Verification items for the finished model (mm, model axes). A direction names the side the tool comes from. Round coordinates to 2 decimals unless told otherwise and drop trailing zeros. Write each loop counter-clockwise with the first axis right and the second up, starting at its lowest first coordinate (ties: lowest second). Pieces come first, ordered by that corner, then holes. Notation, with made-up numbers: M 65,-16.75 L 72,-16.75 A36 ccw 72,19.25 Z; hole C 4,56 d6. An arc over 180 degrees is marked long. Use a Markdown table: item, result. Add a question column.
from build123d import *

# Parameters (mm, degrees)
BOSS_EXTRUDE1_DEPTH = 12
FILLET1_R           = 3
SKETCH4_R           = 0.5
CUT_EXTRUDE3_DEPTH  = 121.732141537
FILLET2_R           = 1
FILLET3_R           = 1
FILLET4_R           = 1
FILLET6_R           = 1
SKETCH2_R           = 2
CUT_EXTRUDE1_DEPTH  = 122.116679281
SKETCH6_R           = 2
CUT_EXTRUDE4_DEPTH  = 8
CUT_EXTRUDE5_DEPTH  = 3.25


with BuildPart() as part:
    # Sketch1 → Boss-Extrude1 (new, symmetric)
    with BuildSketch(Plane(origin=(-107.5, 40, 0), x_dir=(0, 0, -1), z_dir=(1, 0, 0))):
        Polygon((-6.7, -37), (-6.7, -40), (0, -40), (0, -26), (10, -26), (10, -34), (6, -34), (3, -43), (-9.7, -43), (-9.7, -37), align=None)
    extrude(amount=BOSS_EXTRUDE1_DEPTH, both=True)

    # Fillet1
    fillet1_edges = [part.edges().sort_by_distance(p)[0] for p in [
        (-107.5, -3, -3),
        (-107.5, -3, 9.7),
    ]]
    fillet(fillet1_edges, radius=FILLET1_R)

    # Sketch4 → Cut-Extrude3 (cut, through all)
    with BuildSketch(Plane(origin=(0, 0, 0), x_dir=(0, 0, -1), z_dir=(1, 0, 0))):
        with Locations((-6.7, 0)):
            Circle(SKETCH4_R)
        Circle(SKETCH4_R)
    extrude(amount=-CUT_EXTRUDE3_DEPTH, mode=Mode.SUBTRACT)

    # Fillet2
    fillet2_edges = [part.edges().sort_by_distance(p)[0] for p in [
        (-107.5, 0, 6.2),
        (-107.5, 0.5, 6.7),
        (-107.5, 0.5, 0),
        (-107.5, 0, 0.5),
    ]]
    fillet(fillet2_edges, radius=FILLET2_R)

    # Fillet3
    fillet3_edges = [part.edges().sort_by_distance(p)[0] for p in [
        (-107.5, 3, 6.7),
        (-107.5, 3, 9.7),
    ]]
    fillet(fillet3_edges, radius=FILLET3_R)

    # Fillet4
    fillet4_edges = [part.edges().sort_by_distance(p)[0] for p in [
        (-107.5, 14, 0),
        (-107.5, 14, -10),
    ]]
    fillet(fillet4_edges, radius=FILLET4_R)

    # Fillet6
    fillet6_edges = [part.edges().sort_by_distance(p)[0] for p in [
        (-107.5, 6, -10),
        (-107.5, 6, -6),
    ]]
    fillet(fillet6_edges, radius=FILLET6_R)

    # Sketch2 → Cut-Extrude1 (cut, through all)
    with BuildSketch(Plane.XZ.offset(-14)):
        with Locations(Location((-107.5, -5, 0), (0, 0, 41.156184936))):
            Circle(SKETCH2_R)
    extrude(amount=CUT_EXTRUDE1_DEPTH, mode=Mode.SUBTRACT)

    # Sketch6 → Cut-Extrude4 (cut)
    with BuildSketch(Plane(origin=(0, 0, -10), x_dir=(-1, 0, 0), z_dir=(0, 0, -1))):
        with Locations((115.5, 10)):
            Circle(SKETCH6_R)
        with Locations((99.5, 10)):
            Circle(SKETCH6_R)
    extrude(amount=-CUT_EXTRUDE4_DEPTH, mode=Mode.SUBTRACT)

    # Sketch7 → Cut-Extrude5 (cut, symmetric)
    with BuildSketch(Plane(origin=(-107.5, 40, 0), x_dir=(0, 0, -1), z_dir=(1, 0, 0))):
        Polygon((1.88130822, -30.5), (8.38130822, -30.5), (10, -30.5), (10, -43), (8.38130822, -43), (1.88130822, -43), align=None)
    extrude(amount=CUT_EXTRUDE5_DEPTH, both=True, mode=Mode.SUBTRACT)


solid = part.part
1. Access from +Z, -Z, +X, -X, +Y, -Y to the whole of each face (thin tool, end or side, straight path). Record for faces 4 (the flat face through (-107, 3, 8)), 5 (the flat face through (-100, 6, -8)), 6 (the cylindrical face through (-113.502, 10.088, -6.056)).
2. Release check for a two-part mould opening along X. For faces 1 (the flat face through (-115, 10, -2)), 2 (the flat face through (-119.5, 6, -2)), 3 (the cylindrical face through (-107.668, 13.699, -0.285)) record: +X half, -X half, draft (parallel to the pull), parting line (faces both ways), or undercut.
3. Cross-section at B-B on y = 1.5. Enter the section's corners in (x, z).
4. Scan lines: line 1 along X through (y, z) = (13.1, -5); line 2 along Z through (x, y) = (-97, 10.25); line 3 along Y through (x, z) = (-98.75, 4.5). Record each from-to range of solid material in increasing order. Write a range as from..to.
5. Cross-section at A-A on z = -5. Enter the section's corners in (x, y), plus the area to 3 significant figures.
6. Cross-section at D-D on x = -107.5. Enter the section's corners in (y, z).
7. Depth check by flat-ended pin: pin 1 Ø2 at (x, y) = (-107, 2.5) entering from -Z; pin 2 Ø2 at (x, z) = (-108, 3.5) entering from +Y; pin 3 Ø0.7 at (x, z) = (-102, -7.5) entering from -Y; pin 4 Ø10 at (y, z) = (11, 7) entering from -X. Enter the tip coordinate at first touch or a pass-through.
8. Cross-section at C-C on x = -115.5. Enter the section's corners in (y, z), plus the area to 3 significant figures.
Answer:
| question | item | result |
|---|---|---|
| 1 | face 4 | +Z, +X, -X, +Y |
| 1 | face 5 | -Z, +X, -X, -Y |
| 1 | face 6 | -Z |
| 2 | face 1 | undercut |
| 2 | face 2 | -X half |
| 2 | face 3 | draft |
| 3 | outline | M -119.5,-4.5 L -110.75,-4.5 L -110.75,-1.88 L -104.25,-1.88 L -104.25,-4.5 L -95.5,-4.5 L -95.5,0 L -119.5,0 Z; M -119.5,6.7 L -95.5,6.7 L -95.5,9.7 L -119.5,9.7 Z |
| 4 | line 1 | x = -119.5..-109.5, -105.5..-95.5 |
| 4 | line 2 | z = -10..0 |
| 4 | line 3 | y = -3..0 |
| 5 | outline | M -119.5,3 L -110.75,3 L -110.75,9.5 L -109.5,9.5 L -109.5,14 L -119.5,14 Z; M -105.5,9.5 L -104.25,9.5 L -104.25,3 L -95.5,3 L -95.5,14 L -105.5,14 Z; hole C -115.5,10 d4; hole C -99.5,10 d4 |
| 5 | area | 179 mm^2 |
| 6 | outline | M -3,-0.84 A3 ccw -2.81,-1.88 L 9.5,-1.88 L 9.5,-3 L 14,-3 L 14,-1 A1 ccw 13,0 L 1.12,0 A1 ccw 0.37,-0.33 A0.5 cw long -0.33,0.37 A1 ccw 0,1.12 L 0,5.58 A1 ccw -0.33,6.33 A0.5 cw long 0.37,7.03 A1 ccw 1.12,6.7 L 2,6.7 A1 ccw 3,7.7 L 3,8.7 A1 ccw 2,9.7 L 0,9.7 A3 ccw -3,6.7 Z; M 9.5,-10 L 13,-10 A1 ccw 14,-9 L 14,-7 L 9.5,-7 Z |
| 7 | pin 1 | stops at z = -1.88 |
| 7 | pin 2 | stops at y = 0 |
| 7 | pin 3 | stops at y = 6 |
| 7 | pin 4 | passes through |
| 8 | outline | M -3,-0.84 A3 ccw -0.95,-3.68 L 5.32,-5.77 A1 cw 6,-6.72 L 6,-9 A1 ccw 7,-10 L 8,-10 L 8,-2 L 12,-2 L 12,-10 L 13,-10 A1 ccw 14,-9 L 14,-1 A1 ccw 13,0 L 1.12,0 A1 ccw 0.37,-0.33 A0.5 cw long -0.33,0.37 A1 ccw 0,1.12 L 0,5.58 A1 ccw -0.33,6.33 A0.5 cw long 0.37,7.03 A1 ccw 1.12,6.7 L 2,6.7 A1 ccw 3,7.7 L 3,8.7 A1 ccw 2,9.7 L 0,9.7 A3 ccw -3,6.7 Z |
| 8 | area | 121 mm^2 |
